Study the drawing (mm; zero at the part's minimum x, y, z) and answer. Round coordinates to 2 decimals unless told otherwise and drop trailing zeros. Order: outer loops, then holes, each group sorted by start corner. A loop starts at its lowest first (then second) coordinate and runs counter-clockwise, first axis right, second up. Notation, with made-up numbers: (43.5, 75.25) - (75.5, 75.25) arc R18 ccw to (75.5, 84.25) - close; hole circle Ø5 at (30.5, 51.5). An arc over 180 degrees is marked (long way). Use one line per item in the form item = value. Start each with the question number.
Q1. The part is cut by section B-B on z = 39. Determine the outline of the cut face in (x, y), plus the area to 3 significant figures.
Q2. Find the intervals of material crossed by line 1 (X direction, y = 1.3, z = 90); line 2 (Z direction, x = 50, y = 2.1), in increasing order. Write a range as [from, to].
Q3. Given P1, Ø6.5, axis at x = 90, z = 90, coming from the +Y side; P2, Ø6, axis at x = 90, z = 10, coming from the -Y side; P3, Ø3, axis at x = 10, z = 90, coming from the -Y side, each flat-ended and moving along its own axis, determine where each tip first touches the part or whether it passes through.
Q4. For a pull along X with two mould halves and no side action, classify the marked faces 1 and 2 as +X half, -X half, draft (parallel to the pull), parting line (faces both ways), or undercut.
Q5. The part is cut by section A-A on x = 24. Determine the outline of the cut face in (y, z).
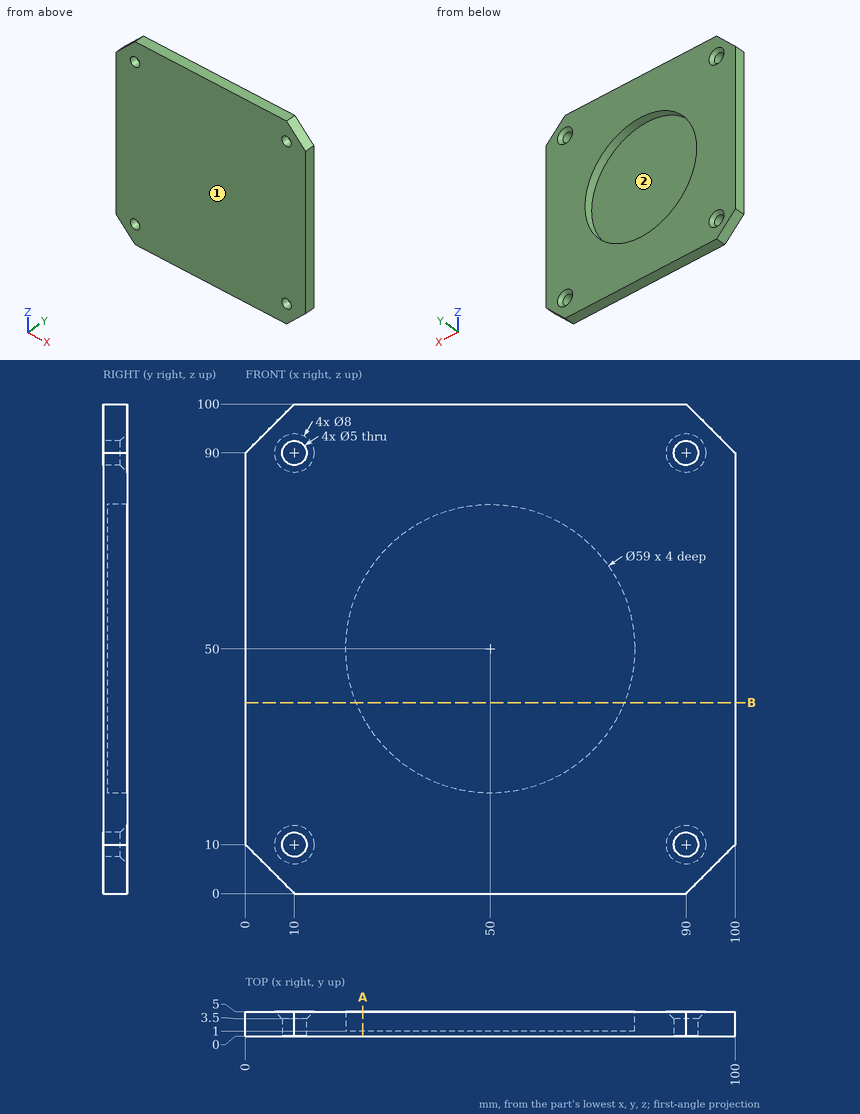
Found:
q1.outline = (0, 0) - (100, 0) - (100, 5) - (77.37, 5) - (77.37, 1) - (22.63, 1) - (22.63, 5) - (0, 5) - close
q1.area = 281 mm²
q2.line_1 = [0, 7.5], [12.5, 87.5], [92.5, 100]
q2.line_2 = [0, 20.5], [79.5, 100]
q3.P1 = 4.25
q3.P2 = 0
q3.P3 = through
q4.face_1 = draft
q4.face_2 = undercut
q5.outline = (0, 0) - (5, 0) - (5, 36.06) - (1, 36.06) - (1, 63.94) - (5, 63.94) - (5, 100) - (0, 100) - close
